Input: part model. Units: mm. Frame: model coordinates. A direction names the side the tool comes from. Round coordinates to 2 decimals unless told otherwise and drop trailing zeros. Order: outer loops, then holes, each group sorted by start corner. A loop starts at its lowest first (then second) coordinate and runs counter-clockwise, first axis right, second up. Notation, with made-up numbers: (29, 45) -> (44, 45) arc R21 ccw to (44, 76) -> close; hole circle Ø5 at (47.5, -8.5). An arc over 180 degrees is marked (long way). Use a Markdown table: item, result.
Autodesk Inventor part; units mm, degrees
ref_plane "YZ Plane" through (0, 0, 0) normal (1, 0, 0) x (0, 1, 0)
ref_plane "XZ Plane" through (0, 0, 0) normal (0, 1, 0) x (-1, 0, 0)
ref_plane "XY Plane" through (0, 0, 0) normal (0, 0, 1) x (1, 0, 0)
sketch "Sketch1" plane through (0, 0, 0) normal (0, 0, 1) x (1, 0, 0)
  line L0 (0, 30.4699) -> (0, 15.4699) construction
  line L1 (4, 30.4699) -> (4, 15.4699)
  line L2 (-4, 15.4699) -> (-4, 30.4699)
  arc A0 (4, 30.4699) -> (-4, 30.4699) centre (0, 30.4699) ccw
  arc A1 (-4, 15.4699) -> (4, 15.4699) centre (0, 15.4699) ccw
  circle A2 centre (0, 0) radius 22.9699 construction
  arc A3 (-18.717, 24.3739) -> (-24.3739, 18.717) centre (-21.5455, 21.5455) ccw
  line L3 (-18.717, 24.3739) -> (-8.1104, 13.7673)
  arc A4 (-13.7673, 8.1104) -> (-8.1104, 13.7673) centre (-10.9389, 10.9389) ccw
  line L4 (-13.7673, 8.1104) -> (-24.3739, 18.717)
  circle A5 centre (0, 0) radius 22.9699 construction
  arc A6 (-30.4699, 4) -> (-30.4699, -4) centre (-30.4699, 0) ccw
  line L5 (-30.4699, 4) -> (-15.4699, 4)
  arc A7 (-15.4699, -4) -> (-15.4699, 4) centre (-15.4699, 0) ccw
  line L6 (-15.4699, -4) -> (-30.4699, -4)
  circle A8 centre (0, 0) radius 22.9699 construction
  arc A9 (-24.3739, -18.7171) -> (-18.717, -24.3739) centre (-21.5455, -21.5455) ccw
  line L7 (-24.3739, -18.7171) -> (-13.7673, -8.1105)
  arc A10 (-8.1104, -13.7673) -> (-13.7673, -8.1105) centre (-10.9389, -10.9389) ccw
  line L8 (-8.1104, -13.7673) -> (-18.717, -24.3739)
  circle A11 centre (0, 0) radius 22.9699 construction
  arc A12 (-4, -30.4699) -> (4, -30.4699) centre (0, -30.4699) ccw
  line L9 (-4, -30.4699) -> (-4, -15.4699)
  arc A13 (4, -15.4699) -> (-4, -15.4699) centre (0, -15.4699) ccw
  line L10 (4, -15.4699) -> (4, -30.4699)
  circle A14 centre (0, 0) radius 22.9699 construction
  arc A15 (18.717, -24.3739) -> (24.3739, -18.7171) centre (21.5455, -21.5455) ccw
  line L11 (18.717, -24.3739) -> (8.1104, -13.7673)
  arc A16 (13.7673, -8.1105) -> (8.1104, -13.7673) centre (10.9389, -10.9389) ccw
  line L12 (13.7673, -8.1105) -> (24.3739, -18.7171)
  circle A17 centre (0, 0) radius 22.9699 construction
  arc A18 (30.4699, -4) -> (30.4699, 4) centre (30.4699, 0) ccw
  line L13 (30.4699, -4) -> (15.4699, -4)
  arc A19 (15.4699, 4) -> (15.4699, -4) centre (15.4699, 0) ccw
  line L14 (15.4699, 4) -> (30.4699, 4)
  circle A20 centre (0, 0) radius 22.9699 construction
  arc A21 (24.3739, 18.717) -> (18.717, 24.3739) centre (21.5455, 21.5455) ccw
  line L15 (24.3739, 18.717) -> (13.7673, 8.1104)
  arc A22 (8.1104, 13.7673) -> (13.7673, 8.1104) centre (10.9389, 10.9389) ccw
  line L16 (8.1104, 13.7673) -> (18.717, 24.3739)
  circle A23 centre (0, 0) radius 22.9699 construction
  line L17 (18.3635, 24.7274) -> (7.7569, 14.1208)
  arc A24 (7.7569, 14.1208) -> (14.1208, 7.7569) centre (10.9389, 10.9389) ccw
  line L18 (14.1208, 7.7569) -> (24.7275, 18.3635)
  arc A25 (24.7275, 18.3635) -> (18.3635, 24.7274) centre (21.5455, 21.5455) ccw
  line L19 (-4.5, 30.4699) -> (-4.5, 15.4699)
  arc A26 (-4.5, 15.4699) -> (4.5, 15.4699) centre (0, 15.4699) ccw
  line L20 (4.5, 15.4699) -> (4.5, 30.4699)
  arc A27 (4.5, 30.4699) -> (-4.5, 30.4699) centre (0, 30.4699) ccw
  line L21 (-7.7569, 14.1208) -> (-18.3635, 24.7274)
  arc A28 (-18.3635, 24.7274) -> (-24.7275, 18.3635) centre (-21.5455, 21.5455) ccw
  line L22 (-24.7275, 18.3635) -> (-14.1208, 7.7569)
  arc A29 (-14.1208, 7.7569) -> (-7.7569, 14.1208) centre (-10.9389, 10.9389) ccw
  line L23 (-15.4699, 4.5) -> (-30.4699, 4.5)
  arc A30 (-30.4699, 4.5) -> (-30.4699, -4.5) centre (-30.4699, 0) ccw
  line L24 (-30.4699, -4.5) -> (-15.4699, -4.5)
  arc A31 (-15.4699, -4.5) -> (-15.4699, 4.5) centre (-15.4699, 0) ccw
  line L25 (15.4699, -4.5) -> (30.4699, -4.5)
  arc A32 (30.4699, -4.5) -> (30.4699, 4.5) centre (30.4699, 0) ccw
  line L26 (30.4699, 4.5) -> (15.4699, 4.5)
  arc A33 (15.4699, 4.5) -> (15.4699, -4.5) centre (15.4699, 0) ccw
  line L27 (-14.1209, -7.7569) -> (-24.7275, -18.3635)
  arc A34 (-24.7275, -18.3635) -> (-18.3635, -24.7275) centre (-21.5455, -21.5455) ccw
  line L28 (-18.3635, -24.7275) -> (-7.7569, -14.1209)
  arc A35 (-7.7569, -14.1209) -> (-14.1209, -7.7569) centre (-10.9389, -10.9389) ccw
  line L29 (-4.5, -15.4699) -> (-4.5, -30.4699)
  arc A36 (-4.5, -30.4699) -> (4.5, -30.4699) centre (0, -30.4699) ccw
  line L30 (4.5, -30.4699) -> (4.5, -15.4699)
  arc A37 (4.5, -15.4699) -> (-4.5, -15.4699) centre (0, -15.4699) ccw
  line L31 (7.7569, -14.1209) -> (18.3635, -24.7275)
  arc A38 (18.3635, -24.7275) -> (24.7275, -18.3635) centre (21.5455, -21.5455) ccw
  line L32 (24.7275, -18.3635) -> (14.1208, -7.7569)
  arc A39 (14.1208, -7.7569) -> (7.7569, -14.1209) centre (10.9389, -10.9389) ccw
  circle A40 centre (0, 0) radius 9
  line L33 (0, 30.9133) -> (0, 15.0265) construction
  line L34 (-7.1776, 30.9133) -> (-7.1776, 15.0265)
  line L35 (7.1776, 15.0265) -> (7.1776, 30.9133)
  arc A41 (7.1776, 30.9133) -> (-7.1776, 30.9133) centre (0, 30.9133) ccw
  arc A42 (-7.1776, 15.0265) -> (7.1776, 15.0265) centre (0, 15.0265) ccw
  arc A43 (-16.7836, 26.9344) -> (-26.9344, 16.7836) centre (-21.859, 21.859) ccw
  line L36 (-5.55, 15.7007) -> (-16.7836, 26.9344)
  arc A44 (-15.7007, 5.5499) -> (-5.55, 15.7007) centre (-10.6253, 10.6253) ccw
  line L37 (-26.9344, 16.7836) -> (-15.7007, 5.5499)
  arc A45 (-30.9133, 7.1776) -> (-30.9133, -7.1777) centre (-30.9133, 0) ccw
  line L38 (-15.0265, 7.1776) -> (-30.9133, 7.1776)
  arc A46 (-15.0265, -7.1777) -> (-15.0265, 7.1776) centre (-15.0265, 0) ccw
  line L39 (-30.9133, -7.1777) -> (-15.0265, -7.1777)
  arc A47 (-26.9344, -16.7837) -> (-16.7836, -26.9344) centre (-21.859, -21.859) ccw
  line L40 (-15.7007, -5.55) -> (-26.9344, -16.7837)
  arc A48 (-5.55, -15.7007) -> (-15.7007, -5.55) centre (-10.6253, -10.6253) ccw
  line L41 (-16.7836, -26.9344) -> (-5.55, -15.7007)
  arc A49 (-7.1776, -30.9133) -> (7.1776, -30.9133) centre (0, -30.9133) ccw
  line L42 (-7.1776, -15.0265) -> (-7.1776, -30.9133)
  arc A50 (7.1776, -15.0265) -> (-7.1776, -15.0265) centre (0, -15.0265) ccw
  line L43 (7.1776, -30.9133) -> (7.1776, -15.0265)
  arc A51 (16.7836, -26.9344) -> (26.9344, -16.7837) centre (21.859, -21.859) ccw
  line L44 (5.55, -15.7007) -> (16.7836, -26.9344)
  arc A52 (15.7007, -5.55) -> (5.55, -15.7007) centre (10.6253, -10.6253) ccw
  line L45 (26.9344, -16.7837) -> (15.7007, -5.55)
  arc A53 (30.9133, -7.1777) -> (30.9133, 7.1776) centre (30.9133, 0) ccw
  line L46 (15.0265, -7.1777) -> (30.9133, -7.1777)
  arc A54 (15.0265, 7.1776) -> (15.0265, -7.1777) centre (15.0265, 0) ccw
  line L47 (30.9133, 7.1776) -> (15.0265, 7.1776)
  arc A55 (26.9344, 16.7836) -> (16.7836, 26.9344) centre (21.859, 21.859) ccw
  line L48 (15.7007, 5.5499) -> (26.9344, 16.7836)
  arc A56 (5.55, 15.7007) -> (15.7007, 5.5499) centre (10.6253, 10.6253) ccw
  line L49 (16.7836, 26.9344) -> (5.55, 15.7007)
  point P0 (0, 0)
  point P1 (0, 22.9699)
  point P2 (-16.2422, 16.2422)
  point P3 (-22.9699, 0)
  point P4 (-16.2422, -16.2422)
  point P5 (0, -22.9699)
  point P6 (16.2422, -16.2422)
  point P7 (22.9699, 0)
  point P8 (16.2422, 16.2422)
  dimension "d2" = 4
  dimension "d3" = 15
  dimension "d4" = 360
  dimension "d6" = 0.5
  dimension "d7" = 0.5
  dimension "d8" = 0.5
  dimension "d9" = 0.5
  dimension "d10" = 0.5
  dimension "d11" = 0.5
  dimension "d12" = 0.5
  dimension "d13" = 0.5
  dimension "d14" = 18
  dimension "d17" = 360
extrude "Extrusion1" add sketch "Sketch1" along normal blind 10 contours L17 A24 A42 L35 L49 A55 L48 L47 A54 L18 A25 | A24 A54 A56 A40 A42 | A42 A56 L49 L35 | A54 L47 L48 A56 | A42 A40 A44 A26 A56 | A56 A33 A52 A54 A40 | A42 A40 | A26 L20 A27 L19 A44 L36 L34 A41 L35 L49 A56 | A40 A56 | L47 A53 L46 L45 A52 A33 L25 A32 L26 A56 L48 | A40 A54 | A44 A42 L34 L36 | A52 L45 L46 A54 | A44 A40 | A40 A44 A46 A29 A42 | A52 A54 A39 A50 A40 | A40 A52 | A29 L21 A28 L22 A46 L38 L37 A43 L36 L34 A42 | L45 A51 L44 L43 A50 A39 L31 A38 L32 A54 L46 | A46 A40 | A40 A46 A48 A31 A44 | A44 L37 L38 A46 | A50 A52 A37 A48 A40 | A40 A50 | A50 L43 L44 A52 | A31 L23 A30 L24 A48 L40 L39 A45 L38 L37 A44 | A52 L44 L43 A49 L42 L41 A48 A37 L29 A36 L30 | A48 A40 | A40 A48 A50 A35 A46 | A46 L39 L40 A48 | A48 L41 L42 A50 | A35 L27 A34 L28 A50 L42 L41 A47 L40 L39 A46
properties part number "location hole mounter"
1) Cut plane D-D on y = -23. Return loops of the section in (x, z).
Results found:
| item | result |
|---|---|
| outline | (-28.95, 0) -> (-25.8, 0) -> (-25.8, 10) -> (-28.95, 10) -> close; (-16.64, 0) -> (-12.85, 0) -> (-12.85, 10) -> (-16.64, 10) -> close; (-7.18, 0) -> (-4.5, 0) -> (-4.5, 10) -> (-7.18, 10) -> close; (4.5, 0) -> (7.18, 0) -> (7.18, 10) -> (4.5, 10) -> close; (12.85, 0) -> (16.64, 0) -> (16.64, 10) -> (12.85, 10) -> close; (25.8, 0) -> (28.95, 0) -> (28.95, 10) -> (25.8, 10) -> close |
2) Cut plane A-A on y = 0. Return loops of the section in (x, z).
Results found:
| item | result |
|---|---|
| outline | (-38.09, 0) -> (-34.97, 0) -> (-34.97, 10) -> (-38.09, 10) -> close; (-10.97, 0) -> (-7.85, 0) -> (-7.85, 10) -> (-10.97, 10) -> close; (7.85, 0) -> (10.97, 0) -> (10.97, 10) -> (7.85, 10) -> close; (34.97, 0) -> (38.09, 0) -> (38.09, 10) -> (34.97, 10) -> close |
3) Line query: L1, parallel to Y at x = -20, z = 4.5; L2, parallel to Y at x = 20.5, z = 7; L3, parallel to Y at x = 12.5, z = 7. Output: solid intervals per line, ascending. Write a range as [from, to].
Results found:
| item | result |
|---|---|
| L1 | y = [-28.79, -25.77], [-13.64, -9.85], [-7.18, -4.5], [4.5, 7.18], [9.85, 13.64], [25.77, 28.79] |
| L2 | y = [-28.91, -25.92], [-14.14, -10.35], [-7.18, -4.5], [4.5, 7.18], [10.35, 14.14], [25.92, 28.91] |
| L3 | y = [-22.65, -18.86], [-6.72, -3.38], [3.38, 6.72], [18.86, 22.65] |
4) Cut plane C-C on x = -32. Return loops of the section in (y, z), and give its area (3 significant figures).
Results found:
| item | result |
|---|---|
| outline | (-7.09, 0) -> (-4.23, 0) -> (-4.23, 10) -> (-7.09, 10) -> close; (4.23, 0) -> (7.09, 0) -> (7.09, 10) -> (4.23, 10) -> close |
| area | 57.3 mm² |
5) Pull-direction query (X, two-part tool) for faces 1 (the flat face through (19.498, -13.134, 4.93)), 2 (the flat face through (24, -7.178, 5)), 3 (the cylindrical face through (38.09, 0.16, 4.93)), 4 (the cylindrical face through (5.6, 5.5, 4.9)); classes: +X half, -X half, draft (parallel to the pull), parting line (faces both ways), or undercut.
Results found:
| item | result |
|---|---|
| face 1 | undercut |
| face 2 | draft |
| face 3 | +X half |
| face 4 | undercut |
6) Pin query (flat end, axial travel): pin 1 Ø5 at (x, z) = (21.5, 3) entering from -Y; pin 2 Ø3 at (x, z) = (-23.5, 6.5) entering from +Y; pin 3 Ø5 at (y, z) = (-27, 7) entering from +X; pin 4 Ø8 at (x, y) = (0, 11) entering from +Z. Return the tip coordinate at first contact, or that it passes through.
Results found:
| item | result |
|---|---|
| pin 1 | stops at y = -29.04 |
| pin 2 | stops at y = 29.04 |
| pin 3 | stops at x = 28.53 |
| pin 4 | stops at z = 10 |
7) Set-up query: faces 5 (the flat face through (12.05, 22.2, 4.93)), 6 (the flat face through (-24, -7.178, 5)), 7 (the flat face through (13.134, 19.498, 4.93)), 8 (the flat face through (-7.178, -24, 5)). Return all of +Z, -Z, +X, -X, +Y, -Y with unobstructed straight access to the full face (end or side cutting, diameter ignored); none if empty.
Results found:
| item | result |
|---|---|
| face 5 | +Z, -Z, +Y |
| face 6 | +Z, -Z, -X |
| face 7 | +Z, -Z |
| face 8 | +Z, -Z, -Y |
